Work out the finished part from the listing and answer in its coordinate system (mm). A direction names the side the tool comes from. Give positions to 0.01 mm unless a question says otherwise; leave off trailing zeros. Write each loop counter-clockwise with the first axis right and the second up, starting at its lowest first coordinate (ties: lowest second). Pieces come first, ordered by that corner, then holes. Notation, with made-up numbers: (89.25, -16) -> (143.25, -16) arc R8 cw to (143.25, -2) -> close; hole circle Ø11 at (34, 16). An arc over 180 degrees is marked (long way). Use a Markdown table: item, result. Add a question column.
Q1. Section B-B, the plane z = 0 is taken. Give the vertices of the cut face in (x, y).
Q2. For faces 1 (the face through (-15, 10, 0)), 2 (the face through (-13, 15, 0)), determine the directions among +Z, -Z, +X, -X, +Y, -Y from which every point of the face is accessible in a straight line to the end or side of a thin tool.
Q3. Consider line 1 (Z direction, x = 0, y = 1.25); line 2 (Y direction, x = 7, z = -6); line 3 (Z direction, x = 0.5, y = 2.5). Determine where each line is inside the solid, lowest interval first.
Q4. For a pull along Z with two mould halves and no side action, classify faces 3 (the face through (-0.54, 2.54, 2.44)), 4 (the face through (0, 0, -4)), 5 (the face through (13.887, 2.465, 10.648)) as pulls with the +Z half, pulls with the -Z half, needs draft (parallel to the pull), parting line crosses it, or undercut.
Q5. This flat-tipped pin is pushed along its axis until it touches: pin 1 Ø4 at (x, z) = (3, 1.5) entering from +Y. Where does it stop, or does it pass through?
Q6. Section D-D, the plane z = -14 is taken. Give the vertices of the cut face in (x, y), plus the area to 3 significant figures.
Q7. Section A-A, the plane x = 0 is taken. Give the vertices of the cut face in (y, z), plus the area to 3 significant figures.
Q8. Section C-C, the plane y = 6.5 is taken. Give the vertices of the cut face in (x, z).
Autodesk Inventor part; units mm, degrees
ref_plane "YZ Plane" through (0, 0, 0) normal (1, 0, 0) x (0, 1, 0)
ref_plane "XZ Plane" through (0, 0, 0) normal (0, 1, 0) x (-1, 0, 0)
ref_plane "XY Plane" through (0, 0, 0) normal (0, 0, 1) x (1, 0, 0)
sketch "Sketch1" plane through (0, 0, 0) normal (0, 1, 0) x (-1, 0, 0)
  circle A0 centre (0, 0) radius 17.5
  dimension "d0" = 35
extrude "Extrusion1" add sketch "Sketch1" along normal blind 5
sketch "Sketch2" plane through (0, 5, 0) normal (0, 1, 0) x (1, 0, 0)
  circle A0 centre (0, 0) radius 12.5 construction
  circle A1 centre (-12.5, 0) radius 2.5
  dimension "d3" = 25
  dimension "d4" = 5
extrude "Extrusion2" add sketch "Sketch2" along normal blind 10
sketch "Sketch3" plane through (0, 5, 0) normal (0, 1, 0) x (1, 0, 0)
  circle A0 centre (0, 0) radius 2.5
  dimension "d7" = 5
extrude "Extrusion3" cut sketch "Sketch3" against normal through all
properties part number "test1"
Result set:
| question | item | result |
|---|---|---|
| 1 | outline | (-17.5, 0) -> (-2.5, 0) -> (-2.5, 5) -> (-10, 5) -> (-10, 15) -> (-15, 15) -> (-15, 5) -> (-17.5, 5) -> close; (2.5, 0) -> (17.5, 0) -> (17.5, 5) -> (2.5, 5) -> close |
| 2 | face 1 | +Y |
| 2 | face 2 | +Z, -Z, +X, -X, +Y |
| 3 | line 1 | z = -17.5 to -2.5, 2.5 to 17.5 |
| 3 | line 2 | y = 0 to 5 |
| 3 | line 3 | z = -17.49 to -2.45, 2.45 to 17.49 |
| 4 | face 3 | undercut |
| 4 | face 4 | needs draft |
| 4 | face 5 | parting line crosses it |
| 5 | pin 1 | stops at y = 5 |
| 6 | outline | (-10.5, 0) -> (10.5, 0) -> (10.5, 5) -> (-10.5, 5) -> close |
| 6 | area | 105 mm2 |
| 7 | outline | (0, -17.5) -> (5, -17.5) -> (5, -2.5) -> (0, -2.5) -> close; (0, 2.5) -> (5, 2.5) -> (5, 17.5) -> (0, 17.5) -> close |
| 7 | area | 150 mm2 |
| 8 | outline | circle Ø5 at (-12.5, 0) |
